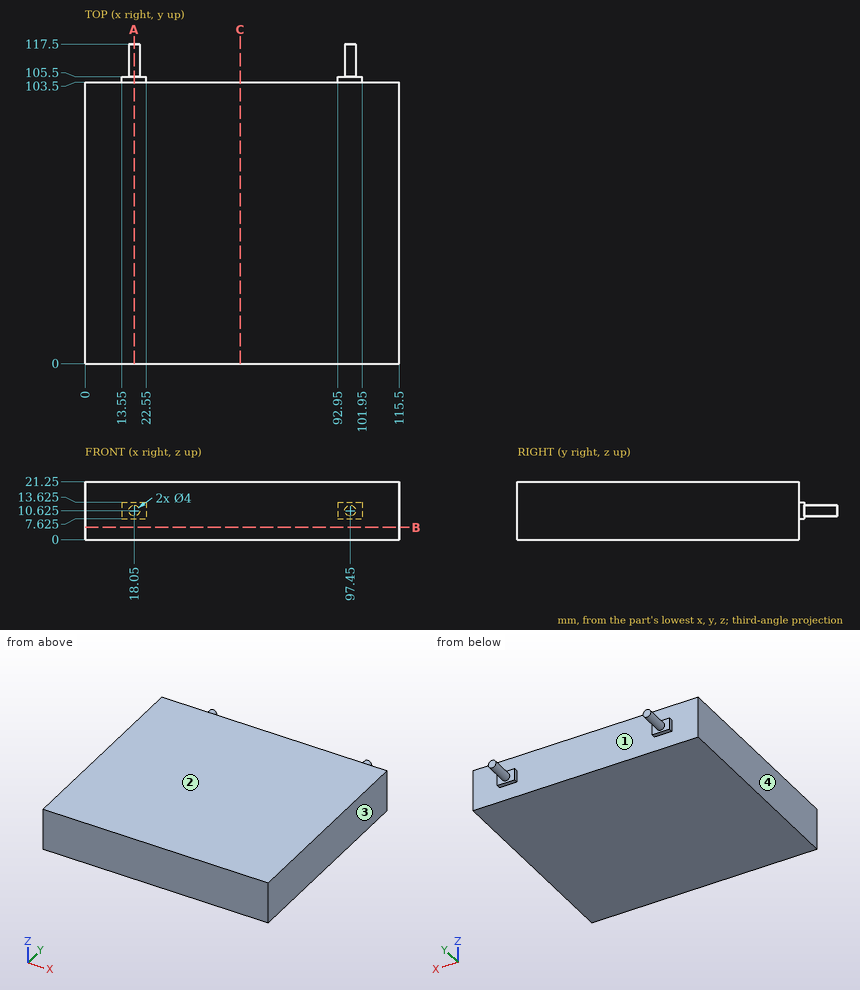
Here's the drawing with two shaded views (mm, measured from the low corner). I have some questions. Give positions to 0.01 mm unless a question says otherwise; leave off trailing zeros. Order: outer loops, then holes, each group sorted by start corner. A loop starts at its lowest first (then second) coordinate and runs counter-clockwise, first axis right, second up. Notation, with made-up numbers: (42, -10.75) - (60, -10.75) arc R29 cw to (60, 19.25) - close; hole circle Ø2 at (33, -34.5). An arc over 180 degrees is marked (long way). Use a Markdown table: item, result. Add a question column.
Q1. I'm going to push flat-ended pins straight in: pin 1 (1 mm diameter, centred on x = 18.5, y = 104.5, fed in from +Z) (3 decimals); pin 2 (1.6 mm diameter, centred on y = 105, z = 11, fed in from -X); pin 3 (0.6 mm diameter, centred on y = 104.5, z = 10.5, fed in from +X). Where does each tip first touch, or does it pass through?
Q2. Please list where this line runs through material, in increasing order: line 1 along Y through (x, z) = (83, 15.5).
Q3. If we section it at C-C on x = 57: Write out the boundary of the cut face in (y, z).
Q4. If we section it at B-B on z = 4.5: Write out the boundary of the cut face in (x, y).
Q5. If we mould it in two halves opening along X, with no side actions, what happens to the marked faces 1, 2, 3 and 4? For each: released by +X, released by -X, zero draft, split by the parting line, or undercut.
Q6. If we section it at A-A on x = 18.05: Write out the boundary of the cut face in (y, z) (3 decimals), plus the area to 3 significant figures.
Answers follow:
| question | item | result |
|---|---|---|
| 1 | pin 1 | stops at z = 13.625 |
| 1 | pin 2 | stops at x = 13.55 |
| 1 | pin 3 | stops at x = 101.95 |
| 2 | line 1 | y = 0 to 103.5 |
| 3 | outline | (0, 0) - (103.5, 0) - (103.5, 21.25) - (0, 21.25) - close |
| 4 | outline | (0, 0) - (115.5, 0) - (115.5, 103.5) - (0, 103.5) - close |
| 5 | face 1 | undercut |
| 5 | face 2 | zero draft |
| 5 | face 3 | released by +X |
| 5 | face 4 | released by -X |
| 6 | outline | (0, 0) - (103.5, 0) - (103.5, 7.625) - (105.5, 7.625) - (105.5, 8.625) - (117.5, 8.625) - (117.5, 12.625) - (105.5, 12.625) - (105.5, 13.625) - (103.5, 13.625) - (103.5, 21.25) - (0, 21.25) - close |
| 6 | area | 2,260 mm^2 |
